Geometry check sheet. Reference: the model listing, model coordinates, mm. A direction names the side the tool comes from. Give positions to 0.01 mm unless a question says otherwise; leave off trailing zeros. Order: outer loops, then holes, each group sorted by start corner. A loop starts at its lowest first (then second) coordinate and runs counter-clockwise, first axis right, second up.
from build123d import *

# Parameters (mm, degrees)
SKETCH_1_W          = 10
SKETCH_1_H          = 10
SKETCH_1_W_2        = 8
SKETCH_1_H_2        = 8
EXTRUDE_1_DEPTH     = 183
SKETCH_2_R          = 2.15
CUT_EXTRUDE_1_DEPTH = 184.341211952


with BuildPart() as part:
    # ｽｹｯﾁ1 → 押し出し-薄板1 (new body)
    with BuildSketch(Plane.XY):
        Rectangle(SKETCH_1_W, SKETCH_1_H)
        Rectangle(SKETCH_1_W_2, SKETCH_1_H_2, mode=Mode.SUBTRACT)
    extrude(amount=EXTRUDE_1_DEPTH)

    # ｽｹｯﾁ2 → ｶｯﾄ - 押し出し1 (cut, through all)
    with BuildSketch(Plane(origin=(5, 0, 0), x_dir=(0, 0, -1), z_dir=(1, 0, 0))):
        with Locations(Location((-128, 0, 0), (0, 0, 90))):
            Circle(SKETCH_2_R)
        with Locations(Location((-108, 0, 0), (0, 0, 90))):
            Circle(SKETCH_2_R)
        with Locations(Location((-148, 0, 0), (0, 0, 90))):
            Circle(SKETCH_2_R)
        with Locations(Location((-178, 0, 0), (0, 0, 90))):
            Circle(SKETCH_2_R)
        with Locations(Location((-78, 0, 0), (0, 0, 90))):
            Circle(SKETCH_2_R)
        with Locations(Location((-5, 0, 0), (0, 0, 90))):
            Circle(SKETCH_2_R)
        with Locations(Location((-25, 0, 0), (0, 0, 90))):
            Circle(SKETCH_2_R)
    extrude(amount=-CUT_EXTRUDE_1_DEPTH, mode=Mode.SUBTRACT)


solid = part.part
Item 1: Draft check along Y on faces 1 (the flat face through (-4.5, 0.1, 183)), 2 (the flat face through (0, -5, 90)), 3 (the flat face through (-4, 0, 90)). Enter one of: released by +Y, released by -Y, zero draft, split by the parting line, or undercut.
Reported:
face 1: zero draft
face 2: released by -Y
face 3: undercut
Item 2: Sectioned sample at A-A (z = 42). Enter the section's corners in (x, y), and give its area (3 significant figures).
Reported:
outline: (-5, -5) - (5, -5) - (5, 5) - (-5, 5) - close; hole (-4, -4) - (4, -4) - (4, 4) - (-4, 4) - close
area: 36.0 mm2
Item 3: Sectioned sample at C-C (x = 0.25). Enter the section's corners in (y, z).
Reported:
outline: (-5, 0) - (-4, 0) - (-4, 183) - (-5, 183) - close; (4, 0) - (5, 0) - (5, 183) - (4, 183) - close
Item 4: Gauge pin test, flat end, axial feed: pin 1 (3 mm diameter, centred on x = -1.5, y = 1, fed in from +Z) (1 decimal). Record the tip position at first contact, or that the pin passes through.
Reported:
pin 1: passes through
Item 5: Set-up check for faces 4 (the cylindrical face through (-4.49, -0.47, 105.9)), 5 (the flat face through (0, -4, 90)): record each of +Z, -Z, +X, -X, +Y, -Y from which the full face is reachable in a straight line by a thin tool's end or side.
Reported:
face 4: +X, -X
face 5: +Z, -Z
Item 6: Sectioned sample at B-B (z = 5). Enter the section's corners in (x, y).
Reported:
outline: (-5, -5) - (5, -5) - (5, -2.15) - (4, -2.15) - (4, -4) - (-4, -4) - (-4, -2.15) - (-5, -2.15) - close; (-5, 2.15) - (-4, 2.15) - (-4, 4) - (4, 4) - (4, 2.15) - (5, 2.15) - (5, 5) - (-5, 5) - close
Item 7: Sectioned sample at D-D (y = 0.25). Give the number of separate pieces and of enclosed holes in the cut face, and give its area (3 significant figures).
Reported:
separate pieces: 16
enclosed holes: 0
area: 306 mm2
Item 8: Scan lines: L1, parallel to X at y = -2.25, z = 18; L2, parallel to Y at x = 4.55, z = 128. Record each from-to range of solid material in increasing order.
Reported:
L1: x = -5 to -4, 4 to 5
L2: y = -5 to -2.15, 2.15 to 5
